Geometry check sheet. Reference: the model listing, model coordinates, mm. A direction names the side the tool comes from. Give positions to 0.01 mm unless a question says otherwise; leave off trailing zeros. Order: outer loops, then holes, each group sorted by start corner. A loop starts at its lowest first (then second) coordinate and runs counter-clockwise, first axis right, second up.
```python
from build123d import *


# Not quite as in the source:
# - a fillet or chamfer that OpenCascade refuses, or shapes differently, is made with other operations: its cross-section is extruded or revolved along the edge and cut away or added


with BuildPart() as f1:
    # F0 (on Front) → F1 (revolve)
    with BuildSketch(Plane.XZ):
        Polygon((0, -16.9278544536), (0, 0), (0, 29), (-9, 29), (-11.5, 0), (-4, 0), (-4, -2.5), (-5.2, -2.5), (-5.2, -5.5), (-2, -8.9278544536), (-2, -16.9278544536), align=None)
    revolve(axis=Axis((0, 0, 14.5), (0, 0, 1)))

    # F2: fillet of radius 3 on 1 edges, made by hand

    # F2_s1 → F2_t2 (revolve)
    with BuildSketch(Plane.XZ):
        with BuildLine():
            ThreePointArc((-4, -0.1), (-4.316718427, -1.4416407865), (-5.2, -2.5))
            Line((-5.2, -2.5), (-5.164, -2.548))
            ThreePointArc((-5.164, -2.548), (-4.6, -2.56), (-4, -2.56))
            Line((-4, -2.56), (-3.94, -2.5))
            Line((-3.94, -2.5), (-3.94, -0.1))
            Line((-3.94, -0.1), (-4, -0.1))
        make_face()
    revolve(axis=Axis((0, 0, -2.5), (0, 0, 1)))


solid = f1.part
```
Q1. Gauge pin test, flat ends, axial feed: P1, Ø1, axis at x = -5, z = 23.5, coming from the +Y side; P2, Ø8, axis at x = 5.5, z = 5, coming from the +Y side; P3, Ø2, axis at y = -2.5, z = 2, coming from the -X side. Record the tip position at first contact, or that the pin passes through.
Q2. Thickness scan on L1, parallel to Z at x = -4.5, y = -1; L2, parallel to Z at x = -4.5, y = 0.5; L3, parallel to Z at x = -7.75, y = -2.75. Record the ranges inside material, lowest first.
Q3. Cross-section at A-A, the plane x = 0. Record the boundary of the cut face in (y, z), and give its area (3 significant figures).
Q4. Cross-section at D-D, the plane z = 21.5. Record the boundary of the cut face in (x, y), and give its area (3 significant figures).
Q5. Access from +Z, -Z, +X, -X, +Y, -Y to the whole of each face (thin tool, end or side, straight path). Record for faces 1 (the face through (0.677, -5.156, -4.021)), 2 (the face through (0, 0, 29)).
Q6. Cross-section at C-C, the plane z = 9. Record the boundary of the cut face in (x, y), and give its area (3 significant figures).
Answers follow:
1. P1: stops at y = 8.34
1. P2: stops at y = 11.06
1. P3: stops at x = -11.25
2. L1: z = -6.13 to -1.91, 0 to 29
2. L2: z = -6.22 to -1.8, 0 to 29
2. L3: z = 0 to 29
3. outline: (-11.5, 0) - (-4, 0) - (-4, -0.1) arc R3 cw to (-5.2, -2.5) - (-5.2, -5.5) - (-2, -8.93) - (-2, -16.93) - (2, -16.93) - (2, -8.93) - (5.2, -5.5) - (5.2, -2.5) arc R3 cw to (4, -0.1) - (4, 0) - (11.5, 0) - (9, 29) - (-9, 29) - close
3. area: 704 mm2
4. outline: circle Ø19.29 at (0, 0)
4. area: 292 mm2
5. face 1: -Z
5. face 2: +Z, +X, -X, +Y, -Y
6. outline: circle Ø21.45 at (0, 0)
6. area: 361 mm2
